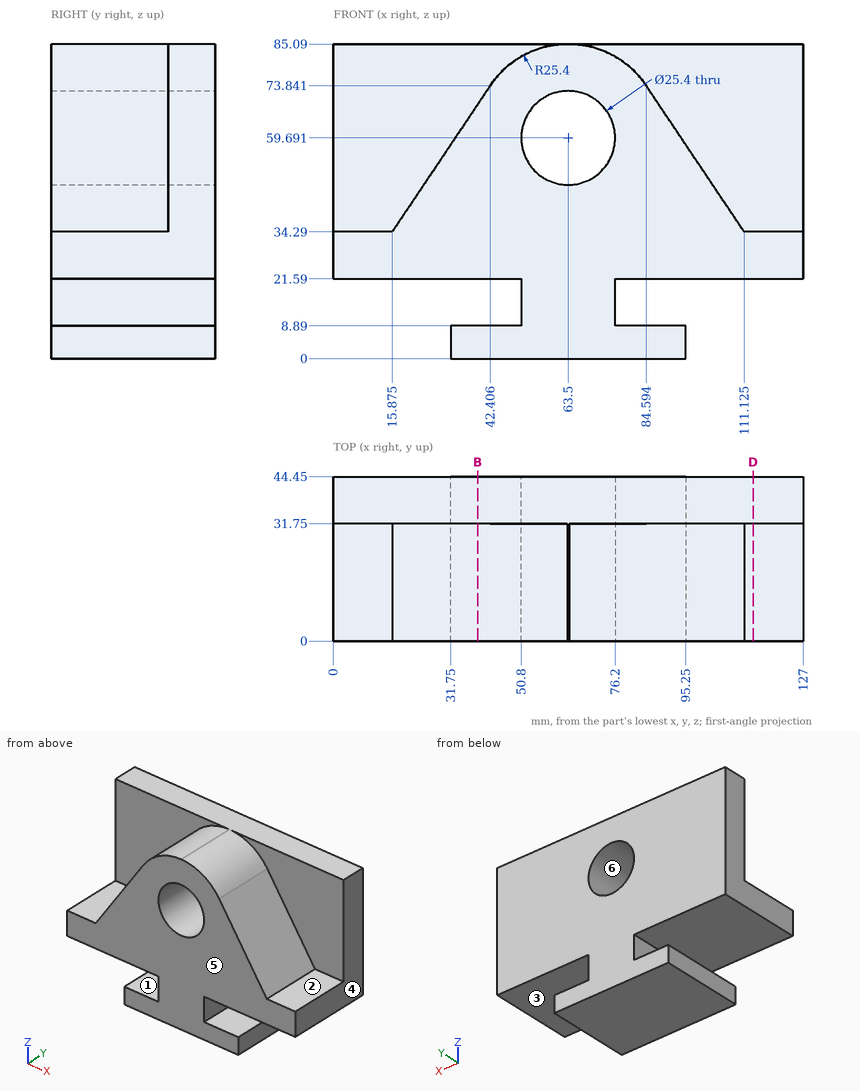
Answer from the drawing. Dimensions are ordinates in mm from the lowest x, y and z of the part. A direction names the side the tool comes from. Coordinates: 2 decimals unless noted, no trailing zeros. Write each loop counter-clockwise with the first axis right and the second up, starting at its lowest first coordinate (ties: lowest second). Pieces come first, ordered by that corner, then holes. Notation, with made-up numbers: M -36.5,39 L 13.5,39 A19 ccw 13.5,61 Z; hole C 5,56 d5. An arc over 180 degrees is marked long. Use one line per item in the form item = value. Start each with the question number.
1. The mould has two halves that part along X. Classify the marked faces 4, 5 and 6: released by +X, released by -X, zero draft, split by the parting line, or undercut.
2. The part is cut by section B-B (x = 39). Give the vertices of the cut face in (y, z), plus the area to 3 significant figures.
3. A tool of negligible diameter and unlimited length cuts with its end or side. For the marked faces 1, 2 and 3, from which of +Z, -Z, +X, -X, +Y, -Y can it reach the whole face along a straight path? Write none if from no direction.
4. Each of these flat-tipped pins is pushed along its axis until it touches: P1, Ø6, axis at x = 49, y = 26, coming from the +Z side; P2, Ø5, axis at x = 119.5, y = 20.5, coming from the +Z side; P3, Ø5, axis at x = 31, y = 15.5, coming from the +Z side (1 decimal). Where does it stop, or does it pass through?
5. The part is cut by section D-D (x = 113.5). Give the vertices of the cut face in (y, z).
6. Straight lines are drawn through the part: probe 1 along Z at (x, y) = (64, 32); probe 2 along Z at (x, y) = (115.5, 36); probe 3 along Z at (x, y) = (13, 24). For each, find the intervals that lie inside material, in ascending order. Write a range as from..to.
Evaluation:
q1.face_4 = released by +X
q1.face_5 = zero draft
q1.face_6 = undercut
q2.outline = M 0,0 L 44.45,0 L 44.45,8.89 L 0,8.89 Z; M 0,21.59 L 44.45,21.59 L 44.45,85.09 L 31.75,85.09 L 31.75,68.76 L 0,68.76 Z
q2.area = 2,700 mm^2
q3.face_1 = -X, +Y, -Y
q3.face_2 = +Z, +X, -Y
q3.face_3 = +X, +Y, -Y
q4.P1 = 82.34
q4.P2 = 34.29
q4.P3 = 60.6
q5.outline = M 0,21.59 L 44.45,21.59 L 44.45,85.09 L 31.75,85.09 L 31.75,34.29 L 0,34.29 Z
q6.probe_1 = 0..47, 72.38..85.09
q6.probe_2 = 21.59..85.09
q6.probe_3 = 21.59..34.29
